Input: part model. Units: mm. Frame: model coordinates. Round coordinates to 2 decimals unless told otherwise and drop trailing zeros. Loops run counter-clockwise (first coordinate to the right, second up) from the corner with the lowest first, then second, coordinate; pieces in that order, holes last. Notation, with made-up numbers: M -7,62 L 37,62 A21 cw 37,70 Z; hole C 58.25,-37 d11. An arc over 180 degrees is marked long. Return JSON: item names as keys, results as strings. Group by question number.
1) Section A-A (z = 0). Output: boundary loops of the cut face in (x, y).
2) Section B-B (y = -70). Output: boundary loops of the cut face in (x, z), plus the area to 3 significant figures.
3) Contact query for flat-ended pins moving along their axis: P1, Ø8, axis at y = 83.5, z = 138, coming from the -X side; P2, Ø1, axis at x = 10, y = -38, coming from the -Z side; P3, Ø5, axis at x = 9.5, z = -103.5, coming from the -Y side; P4, Ø3, axis at x = 2, y = 163.5, coming from the -Z side. Output: stop coordinate, or through.
4) Material intervals for line 1 (Z direction, x = 5.75, y = -105); line 2 (Z direction, x = 11.5, y = -143); line 3 (Z direction, x = 1.5, y = 181), sorted ascending. Write a range as from..to.
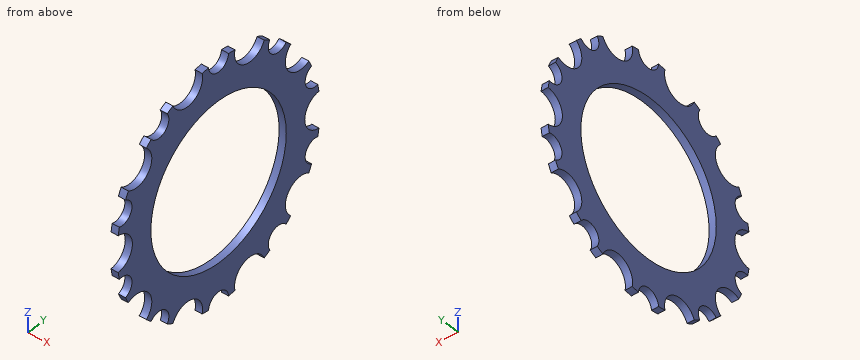
from build123d import *

# Parameters (mm, degrees)
F0_R     = 139.7
F1_DEPTH = 12.7


with BuildPart() as f1:
    # F0 (on Right) → F1 (new body)
    with BuildSketch(Plane.YZ):
        with BuildLine():
            ThreePointArc((20.612464, 208.533759), (0, 188.9125), (-20.612464, 208.533759))
            ThreePointArc((-20.612464, 208.533759), (-27.271164, 207.767866), (-33.901963, 206.789408))
            ThreePointArc((-33.901963, 206.789408), (-54.943222, 169.097849), (-94.120501, 187.223219))
            ThreePointArc((-94.120501, 187.223219), (-100.060053, 184.117322), (-105.897235, 180.823058))
            ThreePointArc((-105.897235, 180.823058), (-111.039981, 152.833423), (-139.248902, 156.591653))
            ThreePointArc((-139.248902, 156.591653), (-144.185722, 152.058147), (-148.975029, 147.369072))
            ThreePointArc((-148.975029, 147.369072), (-143.843222, 104.508218), (-186.192132, 96.144124))
            ThreePointArc((-186.192132, 96.144124), (-189.17173, 90.140219), (-191.957789, 84.044094))
            ThreePointArc((-191.957789, 84.044094), (-179.666464, 58.377173), (-204.696992, 44.836858))
            ThreePointArc((-204.696992, 44.836858), (-206.026236, 38.267384), (-207.144697, 31.658759))
            ThreePointArc((-207.144697, 31.658759), (-177.8, 0), (-207.144697, -31.658759))
            ThreePointArc((-207.144697, -31.658759), (-206.026236, -38.267384), (-204.696992, -44.836858))
            ThreePointArc((-204.696992, -44.836858), (-179.666464, -58.377173), (-191.957789, -84.044094))
            ThreePointArc((-191.957789, -84.044094), (-189.17173, -90.140219), (-186.192132, -96.144124))
            ThreePointArc((-186.192132, -96.144124), (-143.843222, -104.508218), (-148.975029, -147.369072))
            ThreePointArc((-148.975029, -147.369072), (-144.185722, -152.058147), (-139.248902, -156.591653))
            ThreePointArc((-139.248902, -156.591653), (-111.039981, -152.833423), (-105.897235, -180.823058))
            ThreePointArc((-105.897235, -180.823058), (-100.060053, -184.117322), (-94.120501, -187.223219))
            ThreePointArc((-94.120501, -187.223219), (-54.943222, -169.097849), (-33.901963, -206.789408))
            ThreePointArc((-33.901963, -206.789408), (-27.271164, -207.767866), (-20.612464, -208.533759))
            ThreePointArc((-20.612464, -208.533759), (0, -188.9125), (20.612464, -208.533759))
            ThreePointArc((20.612464, -208.533759), (27.271164, -207.767866), (33.901963, -206.789408))
            ThreePointArc((33.901963, -206.789408), (54.943222, -169.097849), (94.120501, -187.223219))
            ThreePointArc((94.120501, -187.223219), (100.060053, -184.117322), (105.897235, -180.823058))
            ThreePointArc((105.897235, -180.823058), (111.039981, -152.833423), (139.248902, -156.591653))
            ThreePointArc((139.248902, -156.591653), (144.185722, -152.058147), (148.975029, -147.369072))
            ThreePointArc((148.975029, -147.369072), (143.843222, -104.508218), (186.192132, -96.144124))
            ThreePointArc((186.192132, -96.144124), (189.17173, -90.140219), (191.957789, -84.044094))
            ThreePointArc((191.957789, -84.044094), (179.666464, -58.377173), (204.696992, -44.836858))
            ThreePointArc((204.696992, -44.836858), (206.026236, -38.267384), (207.144697, -31.658759))
            ThreePointArc((207.144697, -31.658759), (177.8, 0), (207.144697, 31.658759))
            ThreePointArc((207.144697, 31.658759), (206.026236, 38.267384), (204.696992, 44.836858))
            ThreePointArc((204.696992, 44.836858), (179.666464, 58.377173), (191.957789, 84.044094))
            ThreePointArc((191.957789, 84.044094), (189.17173, 90.140219), (186.192132, 96.144124))
            ThreePointArc((186.192132, 96.144124), (143.843222, 104.508218), (148.975029, 147.369072))
            ThreePointArc((148.975029, 147.369072), (144.185722, 152.058147), (139.248902, 156.591653))
            ThreePointArc((139.248902, 156.591653), (111.039981, 152.833423), (105.897235, 180.823058))
            ThreePointArc((105.897235, 180.823058), (100.060053, 184.117322), (94.120501, 187.223219))
            ThreePointArc((94.120501, 187.223219), (54.943222, 169.097849), (33.901963, 206.789408))
            ThreePointArc((33.901963, 206.789408), (27.271164, 207.767866), (20.612464, 208.533759))
        make_face()
        Circle(F0_R, mode=Mode.SUBTRACT)
    extrude(amount=F1_DEPTH)


solid = f1.part
Returned:
{
 "1": {"outline": "M 0,-177.8 L 12.7,-177.8 L 12.7,-139.7 L 0,-139.7 Z; M 0,139.7 L 12.7,139.7 L 12.7,177.8 L 0,177.8 Z"},
 "2": {"outline": "M 0,-167.98 L 12.7,-167.98 L 12.7,-120.9 L 0,-120.9 Z; M 0,120.9 L 12.7,120.9 L 12.7,167.98 L 0,167.98 Z", "area": "1,200 mm^2"},
 "3": {"P1": "stops at x = 0", "P2": "stops at z = -183.01", "P3": "stops at y = -146.8", "P4": "stops at z = -92.33"},
 "4": {"line 1": "z = -181.35..-179.31, -159.74..-92.15, 92.15..159.74, 179.31..181.35", "line 2": "z = -153.17..-140.61, -105.73..105.73, 140.61..153.17", "line 3": "z = -93.56..-74.31, -55.2..-13.89, 13.89..55.2, 74.31..93.56"}
}
